Part model, mm, in its own coordinate system. A direction names the side the tool comes from. Round coordinates to 2 decimals unless told otherwise and drop trailing zeros. Loops run counter-clockwise (first coordinate to the right, second up) from the corner with the lowest first, then second, coordinate; pieces in that order, holes last. Notation, with made-up numbers: M 78.25,66.5 L 86.25,66.5 A9 cw 86.25,82.5 Z; hole C 1,-11 d6. An arc over 180 degrees is marked long. Put each result on its own line as item: value. Start each with the question number.
```python
from build123d import *

# Parameters (mm, degrees)
F0_W        = 40
F0_H        = 40
F1_DEPTH    = 1100
F2_W        = 36
F2_H        = 36
F3_DEPTH    = 1100.001
F4_T1_DEPTH = 245.7346390373


# Not quite as in the source:
# - a fillet or chamfer that OpenCascade refuses, or shapes differently, is made with other operations: its cross-section is extruded or revolved along the edge and cut away or added


with BuildPart() as f1:
    # F0 (on Front) → F1 (new body)
    with BuildSketch(Plane.XZ):
        with Locations((20, 20)):
            Rectangle(F0_W, F0_H)
    extrude(amount=F1_DEPTH)

    # F2 (on face) → F3 (cut, through all)
    with BuildSketch(Plane.XZ.offset(1100)):
        with Locations((20, 20)):
            Rectangle(F2_W, F2_H)
    extrude(amount=-F3_DEPTH, mode=Mode.SUBTRACT)

    # F4: chamfer of 40 on 2 edges, made by hand

    # F4_s2 → F4_t1 (cut)
    with BuildSketch(Plane.YZ.offset(-102.8673195186)):
        Polygon((-1060, 0), (-1100, 40), (-1100, 0), align=None)
        Polygon((-40, 0), (0, 40), (0, 0), align=None)
    extrude(amount=F4_T1_DEPTH, mode=Mode.SUBTRACT)


solid = f1.part
```
1. Wall check: L1, parallel to Z at x = 11, y = -853. Give the ranges that are in metal, low to high.
2. Cut at C-C, the plane x = 14. Give the cut face in (y, z).
3. Mould opens along X. For faces 1 (the flat face through (40, -542, 20)), 2 (the flat face through (20, -543, 0)), 3 (the flat face through (20, -557, 2)) say: released by +X, released by -X, zero draft, split by the parting line, or undercut.
4. Cut at A-A, the plane z = 13.5. Give the cut face in (x, y), and give its area (3 significant figures).
5. Which spindle directions (+Z, -Z, +X, -X, +Y, -Y) get a long thin tool onto all of the face, cutting with end or side? Do faces 4 (the flat face through (39, -1078, 18)), 5 (the flat face through (38, -558, 20)). Say none if no direction does.
6. Cut at B-B, the plane y = -264.5. Give the cut face in (x, z).
Results list:
1. L1: z = 0 to 2, 38 to 40
2. outline: M -1100,40 L -1098,38 L -2,38 L 0,40 Z; M -1062,2 L -1060,0 L -40,0 L -38,2 Z
3. face 1: released by +X
3. face 2: zero draft
3. face 3: undercut
4. outline: M 0,-1073.5 L 2,-1073.5 L 2,-26.5 L 0,-26.5 Z; M 38,-1073.5 L 40,-1073.5 L 40,-26.5 L 38,-26.5 Z
4. area: 4,190 mm^2
5. face 4: -Z, +X, -X, -Y
5. face 5: +Y, -Y
6. outline: M 0,0 L 40,0 L 40,40 L 0,40 Z; hole M 2,2 L 38,2 L 38,38 L 2,38 Z
